```python
from build123d import *

# Parameters (mm, degrees)
F0_R     = 2.75
F1_DEPTH = 6
F2_R     = 11.25
F3_DEPTH = 4


# Not quite as in the source:
# - a fillet or chamfer that OpenCascade refuses, or shapes differently, is made with other operations: its cross-section is extruded or revolved along the edge and cut away or added


with BuildPart() as f1:
    # F0 (on Top) → F1 (new body)
    with BuildSketch(Plane.XY):
        Circle(F0_R)
    extrude(amount=F1_DEPTH)

    # F2 (on face) → F3 (join)
    with BuildSketch(Plane.XY.offset(6)):
        Circle(F2_R)
    extrude(amount=F3_DEPTH)

    # F4: fillet of radius 5 on 1 edges, made by hand

    # F4_s1 → F4_t2 (revolve, cut)
    with BuildSketch(Plane.XZ):
        with BuildLine():
            ThreePointArc((11.25, 6), (9.5132981746, 8.8729833462), (6.3510205144, 10))
            Line((6.3510205144, 10), (11.25, 10))
            Line((11.25, 10), (11.25, 6))
        make_face()
    revolve(axis=Axis((0, 0, 10), (0, 0, 1)), mode=Mode.SUBTRACT)


solid = f1.part
```
Source: CAD feature listing. Evaluate the final solid. Frame: model axes, mm. A direction names the side the tool comes from. Give positions to 0.01 mm unless a question says otherwise; leave off trailing zeros. Order: outer loops, then holes, each group sorted by start corner. A loop starts at its lowest first (then second) coordinate and runs counter-clockwise, first axis right, second up.
(1) Contact query for flat-ended pins moving along their axis: P1, Ø4, axis at x = 3.5, z = 8.5, coming from the +Y side; P2, Ø1.5, axis at y = -1, z = 6.5, coming from the +X side; P3, Ø2, axis at y = -1.5, z = 4, coming from the -X side. Output: stop coordinate, or through.
(2) Section query C-C (z = 4.5). Return the cut outline in (x, y), plus the area to 3 significant figures.
(3) Access query for faces 1 (the face through (-0.596, -2.685, 2.958)), 2 (the face through (0, 0, 0)). Directions: +Z, -Z, +X, -X, +Y, -Y. A direction counts if a zero-diameter tool reaches every point of the face in a straight line with its end or side. Return the directions, or none.
(4) Section query D-D (z = 8). Return the cut outline in (x, y), plus the area to 3 significant figures.
(5) Section query A-A (y = 0). Return the cut outline in (x, z), plus the area to 3 significant figures.
(6) Material intervals for line 1 along Z through (x, y) = (-4.25, -4); line 2 along X through (y, z) = (-6.5, 6.75); line 3 along X through (y, z) = (8.75, 8.5), sorted ascending.
Outcome:
1. P1: stops at y = 10.74
1. P2: stops at x = 11.24
1. P3: stops at x = -2.7
2. outline: circle Ø5.5 at (0, 0)
2. area: 23.8 mm2
3. face 1: -Z
3. face 2: -Z, +X, -X, +Y, -Y
4. outline: circle Ø20.7 at (0, 0)
4. area: 337 mm2
5. outline: (-11.25, 6) - (-2.75, 6) - (-2.75, 0) - (2.75, 0) - (2.75, 6) - (11.25, 6) arc R5 ccw to (6.35, 10) - (-6.35, 10) arc R5 ccw to start
5. area: 113 mm2
6. line 1: z = 6 to 10
6. line 2: x = -8.92 to 8.92
6. line 3: x = -4.68 to 4.68
